```python
from build123d import *

# Parameters (mm, degrees)
SKETCH1_R           = 2.95
BOSS_EXTRUDE1_DEPTH = 1
SKETCH2_R           = 1.35
BOSS_EXTRUDE2_DEPTH = 8
FILLET1_R           = 0.2


with BuildPart() as part:
    # Sketch1 → Boss-Extrude1 (new body)
    with BuildSketch(Plane.XY):
        Circle(SKETCH1_R)
    extrude(amount=BOSS_EXTRUDE1_DEPTH)

    # Sketch2 → Boss-Extrude2 (add)
    with BuildSketch(Plane.XY.offset(1)):
        Circle(SKETCH2_R)
    extrude(amount=BOSS_EXTRUDE2_DEPTH)

    # Fillet1
    fillet1_edges = [part.edges().sort_by_distance(p)[0] for p in [
        (-2.95, 0, 0),
        (-2.95, 0, 1),
        (-1.35, 0, 9),
    ]]
    fillet(fillet1_edges, radius=FILLET1_R)


solid = part.part
```
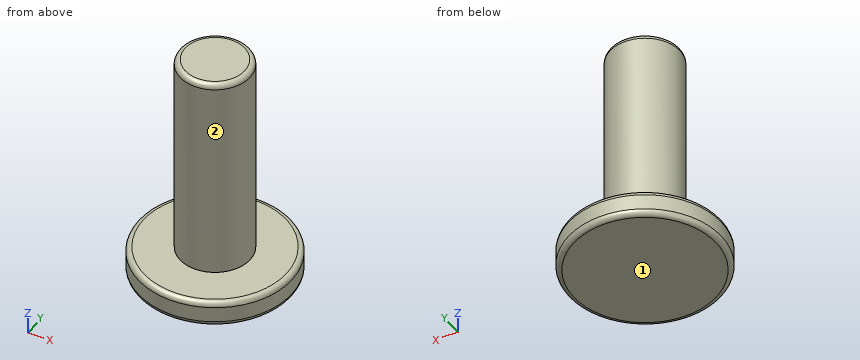
Geometry: final body of the model. Coordinates: model frame, mm. Face numbers are marked on the shaded views. A direction names the side the tool comes from. Coordinates: 2 decimals unless noted, no trailing zeros. Order: outer loops, then holes, each group sorted by start corner. A loop starts at its lowest first (then second) coordinate and runs counter-clockwise, first axis right, second up. Notation, with made-up numbers: (53, 46) - (92, 46) arc R20 cw to (92, 67) - close; hole circle Ø3 at (9, 78). An arc over 180 degrees is marked (long way). Return JSON: item names as keys, results as strings. Group by question number.
1. Pin query (flat end, axial travel): pin 1 (1.5 mm diameter, centred on x = 1, z = 4, fed in from -Y); pin 2 (3 mm diameter, centred on x = -2, y = -1.5, fed in from -Z). Return the tip coordinate at first contact, or that it passes through.
2. Cut plane A-A (y = 0). Output: boundary loops of the cut face in (x, z), plus the area to 3 significant figures.
3. Set-up query: the marked faces 1 and 2. Return all of +Z, -Z, +X, -X, +Y, -Y with unobstructed straight access to the full face (end or side cutting, diameter ignored); none if empty.
4. Material intervals for line 1 along Z through (x, y) = (2.55, -0.6); line 2 along X through (y, z) = (-0.65, 4.75); line 3 along X through (y, z) = (-0.15, 4), sorted ascending. Write a range as [from, to].
5. Cut plane C-C (z = 3.5). Output: boundary loops of the cut face in (x, y), plus the area to 3 significant figures.
Resolved:
{
 "1": {"pin 1": "stops at y = -1.33", "pin 2": "stops at z = 0"},
 "2": {"outline": "(-2.95, 0.2) arc R0.2 ccw to (-2.75, 0) - (2.75, 0) arc R0.2 ccw to (2.95, 0.2) - (2.95, 0.8) arc R0.2 ccw to (2.75, 1) - (1.35, 1) - (1.35, 8.8) arc R0.2 ccw to (1.15, 9) - (-1.15, 9) arc R0.2 ccw to (-1.35, 8.8) - (-1.35, 1) - (-2.75, 1) arc R0.2 ccw to (-2.95, 0.8) - close", "area": "27.4 mm²"},
 "3": {"face 1": "-Z, +X, -X, +Y, -Y", "face 2": "+Z"},
 "4": {"line 1": "z = [0, 1]", "line 2": "x = [-1.18, 1.18]", "line 3": "x = [-1.34, 1.34]"},
 "5": {"outline": "circle Ø2.7 at (0, 0)", "area": "5.73 mm²"}
}
